```python
from build123d import *

# Parameters (mm, degrees)
SKETCH_1_W             = 10
SKETCH_1_H             = 10
EXTRUDE_1_DEPTH        = 22
CUT_EXTRUDE_START      = -5.2
CUT_EXTRUDE_10_DEPTH   = 4.8
SKETCH_14_R            = 1.55
CUT_EXTRUDE_11_DEPTH   = 10
SKETCH_15_W            = 10
SKETCH_15_H            = 9
CUT_EXTRUDE_12_DEPTH   = 4
SKETCH_16_R            = 2.375
CUT_EXTRUDE_13_DEPTH   = 7
CUT_EXTRUDE_14_DEPTH   = 3.3
CHAMFER_1_SIZE         = 0.5
CHAMFER_1_SIZE2        = 0.866025404
CHAMFER_1_PART_2_SIZE  = 0.5
CHAMFER_1_PART_2_SIZE2 = 0.866025404
CHAMFER_1_PART_3_SIZE  = 0.5
CHAMFER_1_PART_3_SIZE2 = 0.866025404
CHAMFER_1_PART_4_SIZE  = 0.5
CHAMFER_1_PART_4_SIZE2 = 0.866025404


with BuildPart() as part:
    # 草图1 → 凸台-拉伸1 (new body)
    with BuildSketch(Plane.XY):
        Rectangle(SKETCH_1_W, SKETCH_1_H)
    extrude(amount=EXTRUDE_1_DEPTH)

    # 草图13 → 切除-拉伸10 (cut)
    with BuildSketch(Plane(origin=(0, 0, 0), x_dir=(-1, 0, 0), z_dir=(0, 0, -1)).offset(CUT_EXTRUDE_START)):
        Polygon((2.6, 1.823001189), (2.6, 6), (-2.6, 6), (-2.6, 1.654219648), (-2.6, -1.5011107), (0, -3.0022214), (2.6, -1.5011107), align=None)
    extrude(amount=-CUT_EXTRUDE_10_DEPTH, mode=Mode.SUBTRACT)

    # 草图14 → 切除-拉伸11 (cut)
    with BuildSketch(Plane(origin=(0, 0, 0), x_dir=(-1, 0, 0), z_dir=(0, 0, -1))):
        Circle(SKETCH_14_R)
    extrude(amount=-CUT_EXTRUDE_11_DEPTH, mode=Mode.SUBTRACT)

    # 草图15 → 切除-拉伸12 (cut)
    with BuildSketch(Plane(origin=(0, 5, 0), x_dir=(1, 0, 0), z_dir=(0, 1, 0))):
        with Locations((0, -17.5)):
            Rectangle(SKETCH_15_W, SKETCH_15_H)
    extrude(amount=-CUT_EXTRUDE_12_DEPTH, mode=Mode.SUBTRACT)

    # 草图16 → 切除-拉伸13 (cut, through all)
    with BuildSketch(Plane(origin=(0, 1, 0), x_dir=(1, 0, 0), z_dir=(0, 1, 0))):
        with Locations((0, -17.5)):
            Circle(SKETCH_16_R)
    extrude(amount=-CUT_EXTRUDE_13_DEPTH, mode=Mode.SUBTRACT)

    # 草图17 → 切除-拉伸14 (cut)
    with BuildSketch(Plane(origin=(0, 0, 0), x_dir=(-1, 0, 0), z_dir=(0, 0, -1))):
        Polygon((5, 5), (2, 5), (5, 2), align=None)
        Polygon((5, -5), (5, -2), (2, -5), align=None)
        Polygon((-5, 5), (-5, 2), (-2, 5), align=None)
        Polygon((-5, -5), (-2, -5), (-5, -2), align=None)
    extrude(amount=-CUT_EXTRUDE_14_DEPTH, mode=Mode.SUBTRACT)

    # 倒角1
    chamfer_1_edges = [part.edges().sort_by_distance(p)[0] for p in [
        (1.55, 0, 5.2),
    ]]
    chamfer_1_side = [part.faces().sort_by_distance(p)[0] for p in [
        (0, 1.701860009, 5.2),
    ]]
    chamfer(chamfer_1_edges, length=CHAMFER_1_SIZE, length2=CHAMFER_1_SIZE2, reference=chamfer_1_side[0])

    # 倒角1 part 2
    chamfer_1_part_2_edges = [part.edges().sort_by_distance(p)[0] for p in [
        (1.55, 0, 0),
    ]]
    chamfer_1_part_2_side = [part.faces().sort_by_distance(p)[0] for p in [
        (-3.4, 3.4, 0),
    ]]
    chamfer(chamfer_1_part_2_edges, length=CHAMFER_1_PART_2_SIZE, length2=CHAMFER_1_PART_2_SIZE2, reference=chamfer_1_part_2_side[0])

    # 倒角1 part 3
    chamfer_1_part_3_edges = [part.edges().sort_by_distance(p)[0] for p in [
        (-2.375, -5, 17.5),
    ]]
    chamfer_1_part_3_side = [part.faces().sort_by_distance(p)[0] for p in [
        (0, -5, 11.383311376),
    ]]
    chamfer(chamfer_1_part_3_edges, length=CHAMFER_1_PART_3_SIZE, length2=CHAMFER_1_PART_3_SIZE2, reference=chamfer_1_part_3_side[0])

    # 倒角1 part 4
    chamfer_1_part_4_edges = [part.edges().sort_by_distance(p)[0] for p in [
        (-2.375, 1, 17.5),
    ]]
    chamfer_1_part_4_side = [part.faces().sort_by_distance(p)[0] for p in [
        (0, 1, 21.86546376),
    ]]
    chamfer(chamfer_1_part_4_edges, length=CHAMFER_1_PART_4_SIZE, length2=CHAMFER_1_PART_4_SIZE2, reference=chamfer_1_part_4_side[0])


solid = part.part
```
Part model, mm, in its own coordinate system. A direction names the side the tool comes from. Round coordinates to 2 decimals unless told otherwise and drop trailing zeros. Order: outer loops, then holes, each group sorted by start corner. A loop starts at its lowest first (then second) coordinate and runs counter-clockwise, first axis right, second up. Notation, with made-up numbers: M 50,-36 L 90,-36 A22 cw 90,-23 Z; hole C 11.25,85 d11. An arc over 180 degrees is marked long. Answer in a Markdown table with one row per item. Add a question column.
Q1. Cut at B-B on y = 3.25. Give the cut face in (x, z).
Q2. Cut at C-C on z = 2.25. Give the cut face in (x, y), and give its area (3 significant figures).
Q3. Cut at A-A on z = 17.5. Give the cut face in (x, y) (3 decimals).
Q4. Pin check, flat tips, straight feed: pin 1 (0.9 mm diameter, centred on x = -4, y = -4, fed in from -Z); pin 2 (6 mm diameter, centred on x = 0, z = 17.5, fed in from +Y); pin 3 (2 mm diameter, centred on x = 0, y = 3, fed in from +Z). Stop position of each tip, or through.
Q5. Cut at D-D on x = 4. Give the cut face in (y, z), and give its area (3 significant figures).
Q6. Wall check: L1, parallel to X at y = -1.25, z = 7.25; L2, parallel to Y at x = 0, z = 3.6; L3, parallel to X at y = -2.9, z = 17.5 (3 decimals). Give the ranges that are in metal, low to high. Write a range as from..to.
Q7. 3-axis set-ups, long thin cutter, end or side, ignore diameter. For faces 4 (the face through (4, 3, 2)), 5 (the face through (2, 1, 15)), 6 (the face through (4, -4, 3.3)), 7 (the face through (0, 3, 5.2)), 8 (the face through (-3, 4, 2)): which of +Z, -Z, +X, -X, +Y, -Y reach the whole face in a straight line?
Q8. Mould opens along Y. For faces 1 (the face through (2.2, 0.1, 0)), 2 (the face through (0, 5, 5)), 3 (the face through (-0.715, -1.375, 2.576)) say: +Y half, -Y half, draft (parallel to the pull), parting line (faces both ways), or undercut.
Established:
| question | item | result |
|---|---|---|
| 1 | outline | M -5,3.3 L -3.75,3.3 L -3.75,0 L 3.75,0 L 3.75,3.3 L 5,3.3 L 5,13 L -5,13 Z; hole M -2.6,5.2 L 2.6,5.2 L 2.6,10 L -2.6,10 Z |
| 2 | outline | M -5,-2 L -2,-5 L 2,-5 L 5,-2 L 5,2 L 2,5 L -2,5 L -5,2 Z; hole C 0,0 d3.1 |
| 2 | area | 74.5 mm2 |
| 3 | outline | M -5,-5 L -2.875,-5 L -2.375,-4.134 L -2.375,0.134 L -2.875,1 L -5,1 Z; M 2.375,-4.134 L 2.875,-5 L 5,-5 L 5,1 L 2.875,1 L 2.375,0.134 Z |
| 4 | pin 1 | stops at z = 3.3 |
| 4 | pin 2 | stops at y = 1 |
| 4 | pin 3 | stops at z = 13 |
| 5 | outline | M -5,3.3 L -3,3.3 L -3,0 L 3,0 L 3,3.3 L 5,3.3 L 5,13 L 1,13 L 1,22 L -5,22 Z |
| 5 | area | 171 mm2 |
| 6 | L1 | x = -5..-2.6, 2.6..5 |
| 6 | L2 | y = -5..-1.55, 1.55..5 |
| 6 | L3 | x = -5..-2.375, 2.375..5 |
| 7 | face 4 | -Z, +X, +Y |
| 7 | face 5 | +Z, +X, -X, +Y |
| 7 | face 6 | -Z, +X, -Y |
| 7 | face 7 | +Y |
| 7 | face 8 | -Z, -X, +Y |
| 8 | face 1 | draft |
| 8 | face 2 | +Y half |
| 8 | face 3 | undercut |
